Check sheet for the modelled part. Datum: model origin and axes. Units: mm. Round coordinates to 2 decimals unless told otherwise and drop trailing zeros. Order: outer loops, then holes, each group sorted by start corner. A loop starts at its lowest first (then second) coordinate and runs counter-clockwise, first axis right, second up. Notation, with made-up numbers: (-4.75, 87) -> (0.25, 87) arc R24 cw to (0.25, 121) -> close; hole circle Ø7 at (85.25, 34). An arc over 180 degrees is marked (long way). Answer in a Markdown table with one row per item.
```python
from build123d import *

# Parameters (mm, degrees)
SALIENTE_EXTRUIR1_DEPTH = 0.1


with BuildPart() as part:
    # Model → Saliente-Extruir1 (new body)
    with BuildSketch(Plane.XY):
        with BuildLine():
            Line((14.520286295, 27.479285465), (30.020286295, 27.479285465))
            Line((30.020286295, 27.479285465), (30.995526762, 27.479285465))
            Line((30.995526762, 27.479285465), (46.520286295, 27.479285465))
            Line((46.520286295, 27.479285465), (46.520286295, -0.733231614))
            Line((46.520286295, -0.733231614), (51.471061016, 23.659269995))
            ThreePointArc((51.471061016, 23.659269995), (55.350844588, 27.68663731), (60.617590106, 25.806796971))
            ThreePointArc((60.617590106, 25.806796971), (57.96035452, 32.1636369), (51.115344163, 32.948587895))
            ThreePointArc((51.115344163, 32.948587895), (50.436854059, 32.782110426), (49.742499175, 32.859148502))
            Line((49.742499175, 32.859148502), (43.04104749, 34.830163703))
            ThreePointArc((43.04104749, 34.830163703), (42.188067529, 35.337786997), (41.684191584, 36.192985954))
            Line((41.684191584, 36.192985954), (39.61828219, 42.24428199))
            ThreePointArc((39.61828219, 42.24428199), (46.085307041, 47.434632953), (51.291287848, 53.889082378))
            ThreePointArc((51.291287848, 53.889082378), (57.354652208, 70.765408557), (54.99199246, 88.541589574))
            ThreePointArc((54.99199246, 88.541589574), (53.468862534, 91.179848081), (51.222076914, 93.237100398))
            ThreePointArc((51.222076914, 93.237100398), (45.021608732, 96.446811627), (38.244470176, 98.125634086))
            ThreePointArc((38.244470176, 98.125634086), (30.716762072, 98.976544856), (23.183606681, 98.175290659))
            ThreePointArc((23.183606681, 98.175290659), (16.202528521, 96.493815521), (9.804335921, 93.234069768))
            ThreePointArc((9.804335921, 93.234069768), (7.557851393, 91.176488668), (6.035107577, 88.538007288))
            ThreePointArc((6.035107577, 88.538007288), (3.675049302, 70.761480699), (9.740883355, 53.886042041))
            ThreePointArc((9.740883355, 53.886042041), (14.947788987, 47.432374192), (21.41554616, 42.242979995))
            Line((21.41554616, 42.242979995), (19.35050339, 36.191373826))
            ThreePointArc((19.35050339, 36.191373826), (18.846750914, 35.336102135), (17.993844246, 34.828355703))
            Line((17.993844246, 34.828355703), (11.292677181, 32.856373051))
            ThreePointArc((11.292677181, 32.856373051), (10.598333426, 32.779234734), (9.919819295, 32.945614249))
            ThreePointArc((9.919819295, 32.945614249), (3.074922331, 32.159675066), (0.418604493, 25.802451585))
            ThreePointArc((0.418604493, 25.802451585), (5.241056245, 27.958298833), (9.263373954, 24.534167044))
            Line((9.263373954, 24.534167044), (14.520286295, -0.733231614))
            Line((14.520286295, -0.733231614), (14.520286295, 27.479285465))
        make_face()
        with BuildLine():
            ThreePointArc((28.153211973, 61.525805428), (26.284358187, 74.589260971), (15.542822199, 82.255152297))
            ThreePointArc((15.542822199, 82.255152297), (11.073088945, 83.602659269), (6.85998466, 85.613639796))
            ThreePointArc((6.85998466, 85.613639796), (7.253715162, 72.399202471), (16.442622696, 62.89444809))
            ThreePointArc((16.442622696, 62.89444809), (22.215756006, 61.507125455), (28.153211973, 61.525805428))
        make_face(mode=Mode.SUBTRACT)
        with BuildLine():
            ThreePointArc((32.866716238, 61.523161648), (38.809998945, 61.505477347), (44.588230247, 62.896507568))
            ThreePointArc((44.588230247, 62.896507568), (53.775746714, 72.402606594), (54.167543352, 85.617101397))
            ThreePointArc((54.167543352, 85.617101397), (49.954733408, 83.605504327), (45.485197402, 82.257343249))
            ThreePointArc((45.485197402, 82.257343249), (34.736372016, 74.592110583), (32.866716238, 61.523161648))
        make_face(mode=Mode.SUBTRACT)
    extrude(amount=SALIENTE_EXTRUIR1_DEPTH)


solid = part.part
```
(1) Section check B-B on x = 48. Record the boundary of the cut face in (y, z), plus the area to 3 significant figures.
Solutions:
| item | result |
|---|---|
| outline | (6.56, 0) -> (33.37, 0) -> (33.37, 0.1) -> (6.56, 0.1) -> close; (49.49, 0) -> (64.95, 0) -> (64.95, 0.1) -> (49.49, 0.1) -> close; (82.92, 0) -> (95.13, 0) -> (95.13, 0.1) -> (82.92, 0.1) -> close |
| area | 5.45 mm^2 |
(2) Scan lines: probe 1 along Y at (x, z) = (45, 0.05); probe 2 along Y at (x, z) = (17, 0.05); probe 3 along Y at (x, z) = (35.5, 0.05). Record each from-to range of solid material in increasing order. Write a range as from..to.
Solutions:
| item | result |
|---|---|
| probe 1 | 27.48..34.25, 46.39..63.09, 82.14..96.45 |
| probe 2 | 27.48..34.54, 45.53..62.7, 81.87..96.78 |
| probe 3 | 27.48..61.34, 75.74..98.63 |
(3) Section check D-D on y = 70. Record the boundary of the cut face in (x, z).
Solutions:
| item | result |
|---|---|
| outline | (3.76, 0) -> (8.48, 0) -> (8.48, 0.1) -> (3.76, 0.1) -> close; (28.21, 0) -> (32.81, 0) -> (32.81, 0.1) -> (28.21, 0.1) -> close; (52.55, 0) -> (57.27, 0) -> (57.27, 0.1) -> (52.55, 0.1) -> close |
(4) Section check A-A on z = 0.05. Give the number of separate pieces and of enclosed holes in the cut face, plus the area to 3 significant figures.
Solutions:
| item | result |
|---|---|
| separate pieces | 1 |
| enclosed holes | 2 |
| area | 2,480 mm^2 |
(5) Section check C-C on y = 10. Record the boundary of the cut face in (x, z).
Solutions:
| item | result |
|---|---|
| outline | (12.29, 0) -> (14.52, 0) -> (14.52, 0.1) -> (12.29, 0.1) -> close; (46.52, 0) -> (48.7, 0) -> (48.7, 0.1) -> (46.52, 0.1) -> close |
